```python
from build123d import *

# Parameters (mm, degrees)
SKETCH1_W             = 93.653112922
SKETCH1_H             = 50
BOSS_EXTRUDE1_DEPTH   = 2.8575
SKETCH3_W             = 23.386037641
SKETCH3_H             = 4.318
BOSS_EXTRUDE2_DEPTH   = 2.8575
CUT_EXTRUDE1_REACH    = 4.857
SKETCH4_W             = 4.572
SKETCH4_H             = 14.7575
SKETCH4_H_2           = 6.0325
CUT_EXTRUDE2_REACH    = 4.857
SKETCH5_W             = 20.574
SKETCH5_H             = 2.9845
SKETCH6_R             = 0.635
CUT_EXTRUDE3_DEPTH    = 0.127
CHAMFER1_SIZE         = 0.762
CHAMFER1_SIZE2        = 1.319822715
CHAMFER1_PART_2_SIZE  = 0.762
CHAMFER1_PART_2_SIZE2 = 1.319822715
CHAMFER1_PART_3_SIZE  = 0.762
CHAMFER1_PART_3_SIZE2 = 1.319822715
CHAMFER1_PART_4_SIZE  = 0.762
CHAMFER1_PART_4_SIZE2 = 1.319822715
CHAMFER2_SIZE         = 0.762
CHAMFER2_SIZE2        = 1.319822715
CHAMFER2_PART_2_SIZE  = 0.762
CHAMFER2_PART_2_SIZE2 = 1.319822715
CHAMFER2_PART_3_SIZE  = 0.762
CHAMFER2_PART_3_SIZE2 = 1.319822715
CHAMFER2_PART_4_SIZE  = 0.762
CHAMFER2_PART_4_SIZE2 = 1.319822715
FILLET1_R             = 0.762


with BuildPart() as part:
    # Sketch1 → Boss-Extrude1 (new body)
    with BuildSketch(Plane(origin=(0, 0, 0), x_dir=(1, 0, 0), z_dir=(0, 1, 0))):
        Rectangle(SKETCH1_W, SKETCH1_H)
    extrude(amount=BOSS_EXTRUDE1_DEPTH)

    # Sketch3 → Boss-Extrude2 (add)
    with BuildSketch(Plane.XZ):
        with Locations((-22.751037641, 27.159)):
            Rectangle(SKETCH3_W, SKETCH3_H)
        with Locations((22.751037641, 27.159)):
            Rectangle(SKETCH3_W, SKETCH3_H)
    extrude(amount=-BOSS_EXTRUDE2_DEPTH)

    # Sketch4 → Cut-Extrude1 (cut, up to next)
    with BuildSketch(Plane(origin=(0, 2.8575, 0), x_dir=(1, 0, 0), z_dir=(0, 1, 0)), mode=Mode.PRIVATE) as cut_extrude1_sk1:
        with Locations((44.540556461, 17.62125)):
            Rectangle(SKETCH4_W, SKETCH4_H)
    cut_extrude1_tool1 = extrude(cut_extrude1_sk1.sketch, amount=-CUT_EXTRUDE1_REACH, mode=Mode.PRIVATE) & part.part
    add(cut_extrude1_tool1.solids().sort_by_distance((44.540556, 2.8575, -17.62125))[0], mode=Mode.SUBTRACT)
    # Sketch4 → Cut-Extrude1 (cut, up to next)
    with BuildSketch(Plane(origin=(0, 2.8575, 0), x_dir=(1, 0, 0), z_dir=(0, 1, 0)), mode=Mode.PRIVATE) as cut_extrude1_sk2:
        with Locations((44.540556461, -21.98375)):
            Rectangle(SKETCH4_W, SKETCH4_H_2)
    cut_extrude1_tool2 = extrude(cut_extrude1_sk2.sketch, amount=-CUT_EXTRUDE1_REACH, mode=Mode.PRIVATE) & part.part
    add(cut_extrude1_tool2.solids().sort_by_distance((44.540556, 2.8575, 21.98375))[0], mode=Mode.SUBTRACT)
    # Sketch4 → Cut-Extrude1 (cut, up to next)
    with BuildSketch(Plane(origin=(0, 2.8575, 0), x_dir=(1, 0, 0), z_dir=(0, 1, 0)), mode=Mode.PRIVATE) as cut_extrude1_sk3:
        with Locations((-44.540556461, 17.62125)):
            Rectangle(SKETCH4_W, SKETCH4_H)
    cut_extrude1_tool3 = extrude(cut_extrude1_sk3.sketch, amount=-CUT_EXTRUDE1_REACH, mode=Mode.PRIVATE) & part.part
    add(cut_extrude1_tool3.solids().sort_by_distance((-44.540556, 2.8575, -17.62125))[0], mode=Mode.SUBTRACT)
    # Sketch4 → Cut-Extrude1 (cut, up to next)
    with BuildSketch(Plane(origin=(0, 2.8575, 0), x_dir=(1, 0, 0), z_dir=(0, 1, 0)), mode=Mode.PRIVATE) as cut_extrude1_sk4:
        with Locations((-44.540556461, -21.98375)):
            Rectangle(SKETCH4_W, SKETCH4_H_2)
    cut_extrude1_tool4 = extrude(cut_extrude1_sk4.sketch, amount=-CUT_EXTRUDE1_REACH, mode=Mode.PRIVATE) & part.part
    add(cut_extrude1_tool4.solids().sort_by_distance((-44.540556, 2.8575, 21.98375))[0], mode=Mode.SUBTRACT)

    # Sketch5 → Cut-Extrude2 (cut, up to next)
    with BuildSketch(Plane.XZ, mode=Mode.PRIVATE) as cut_extrude2_sk1:
        with Locations((22.225, -18.74525)):
            Rectangle(SKETCH5_W, SKETCH5_H)
    cut_extrude2_tool1 = extrude(cut_extrude2_sk1.sketch, amount=-CUT_EXTRUDE2_REACH, mode=Mode.PRIVATE) & part.part
    add(cut_extrude2_tool1.solids().sort_by_distance((22.225, 0, -18.74525))[0], mode=Mode.SUBTRACT)
    # Sketch5 → Cut-Extrude2 (cut, up to next)
    with BuildSketch(Plane.XZ, mode=Mode.PRIVATE) as cut_extrude2_sk2:
        with Locations((-22.225, -18.74525)):
            Rectangle(SKETCH5_W, SKETCH5_H)
    cut_extrude2_tool2 = extrude(cut_extrude2_sk2.sketch, amount=-CUT_EXTRUDE2_REACH, mode=Mode.PRIVATE) & part.part
    add(cut_extrude2_tool2.solids().sort_by_distance((-22.225, 0, -18.74525))[0], mode=Mode.SUBTRACT)

    # Sketch6 → Cut-Extrude3 (cut)
    with BuildSketch(Plane.XZ):
        with Locations((-25.799037641, 26.778)):
            Circle(SKETCH6_R)
        with Locations((-23.767037641, 26.778)):
            Circle(SKETCH6_R)
        with Locations((-21.735037641, 26.778)):
            Circle(SKETCH6_R)
        with Locations((-19.703037641, 26.778)):
            Circle(SKETCH6_R)
        with Locations((19.703037641, 26.778)):
            Circle(SKETCH6_R)
        with Locations((21.735037641, 26.778)):
            Circle(SKETCH6_R)
        with Locations((23.767037641, 26.778)):
            Circle(SKETCH6_R)
        with Locations((25.799037641, 26.778)):
            Circle(SKETCH6_R)
        with Locations((44.286556461, 4.3625)):
            Circle(SKETCH6_R)
        with Locations((-44.286556461, 7.4105)):
            Circle(SKETCH6_R)
        with Locations((-44.286556461, 5.3785)):
            Circle(SKETCH6_R)
        with Locations((-44.286556461, 3.3465)):
            Circle(SKETCH6_R)
        with Locations((-44.286556461, 1.3145)):
            Circle(SKETCH6_R)
    extrude(amount=-CUT_EXTRUDE3_DEPTH, mode=Mode.SUBTRACT)

    # Chamfer1
    chamfer1_edges = [part.edges().sort_by_distance(p)[0] for p in [
        (-34.444056461, 1.42875, 29.318),
    ]]
    chamfer1_side = [part.faces().sort_by_distance(p)[0] for p in [
        (-22.751037641, 1.42875, 29.318),
    ]]
    chamfer(chamfer1_edges, length=CHAMFER1_SIZE, length2=CHAMFER1_SIZE2, reference=chamfer1_side[0])

    # Chamfer1 part 2
    chamfer1_part_2_edges = [part.edges().sort_by_distance(p)[0] for p in [
        (11.05801882, 1.42875, 29.318),
    ]]
    chamfer1_part_2_side = [part.faces().sort_by_distance(p)[0] for p in [
        (22.751037641, 1.42875, 29.318),
    ]]
    chamfer(chamfer1_part_2_edges, length=CHAMFER1_PART_2_SIZE, length2=CHAMFER1_PART_2_SIZE2, reference=chamfer1_part_2_side[0])

    # Chamfer1 part 3
    chamfer1_part_3_edges = [part.edges().sort_by_distance(p)[0] for p in [
        (-46.826556461, 1.42875, 18.9675),
    ]]
    chamfer1_part_3_side = [part.faces().sort_by_distance(p)[0] for p in [
        (-46.826556461, 1.42875, 4.3625),
    ]]
    chamfer(chamfer1_part_3_edges, length=CHAMFER1_PART_3_SIZE, length2=CHAMFER1_PART_3_SIZE2, reference=chamfer1_part_3_side[0])

    # Chamfer1 part 4
    chamfer1_part_4_edges = [part.edges().sort_by_distance(p)[0] for p in [
        (46.826556461, 1.42875, -10.2425),
    ]]
    chamfer1_part_4_side = [part.faces().sort_by_distance(p)[0] for p in [
        (46.826556461, 1.42875, 4.3625),
    ]]
    chamfer(chamfer1_part_4_edges, length=CHAMFER1_PART_4_SIZE, length2=CHAMFER1_PART_4_SIZE2, reference=chamfer1_part_4_side[0])

    # Chamfer2
    chamfer2_edges = [part.edges().sort_by_distance(p)[0] for p in [
        (-11.05801882, 1.42875, 29.318),
    ]]
    chamfer2_side = [part.faces().sort_by_distance(p)[0] for p in [
        (-22.370037641, 1.42875, 29.318),
    ]]
    chamfer(chamfer2_edges, length=CHAMFER2_SIZE, length2=CHAMFER2_SIZE2, reference=chamfer2_side[0])

    # Chamfer2 part 2
    chamfer2_part_2_edges = [part.edges().sort_by_distance(p)[0] for p in [
        (34.444056461, 1.42875, 29.318),
    ]]
    chamfer2_part_2_side = [part.faces().sort_by_distance(p)[0] for p in [
        (23.132037641, 1.42875, 29.318),
    ]]
    chamfer(chamfer2_part_2_edges, length=CHAMFER2_PART_2_SIZE, length2=CHAMFER2_PART_2_SIZE2, reference=chamfer2_part_2_side[0])

    # Chamfer2 part 3
    chamfer2_part_3_edges = [part.edges().sort_by_distance(p)[0] for p in [
        (46.826556461, 1.42875, 18.9675),
    ]]
    chamfer2_part_3_side = [part.faces().sort_by_distance(p)[0] for p in [
        (46.826556461, 1.42875, 4.7435),
    ]]
    chamfer(chamfer2_part_3_edges, length=CHAMFER2_PART_3_SIZE, length2=CHAMFER2_PART_3_SIZE2, reference=chamfer2_part_3_side[0])

    # Chamfer2 part 4
    chamfer2_part_4_edges = [part.edges().sort_by_distance(p)[0] for p in [
        (-46.826556461, 1.42875, -10.2425),
    ]]
    chamfer2_part_4_side = [part.faces().sort_by_distance(p)[0] for p in [
        (-46.826556461, 1.42875, 3.9815),
    ]]
    chamfer(chamfer2_part_4_edges, length=CHAMFER2_PART_4_SIZE, length2=CHAMFER2_PART_4_SIZE2, reference=chamfer2_part_4_side[0])

    # Fillet1
    fillet1_edges = [part.edges().sort_by_distance(p)[0] for p in [
        (11.938, 1.42875, -20.2375),
        (11.938, 1.42875, -17.253),
        (32.512, 1.42875, -17.253),
        (32.512, 1.42875, -20.2375),
        (-32.512, 1.42875, -20.2375),
        (-32.512, 1.42875, -17.253),
        (-11.938, 1.42875, -17.253),
        (-11.938, 1.42875, -20.2375),
    ]]
    fillet(fillet1_edges, radius=FILLET1_R)


solid = part.part
```
The listing builds one solid part. Answer for the finished solid, in the listing's coordinates (mm). A direction names the side the tool comes from. Round coordinates to 2 decimals unless told otherwise and drop trailing zeros. Loops run counter-clockwise (first coordinate to the right, second up) from the corner with the lowest first, then second, coordinate; pieces in that order, holes last. Notation, with made-up numbers: (10, -34) - (31, -34) arc R7 cw to (31, -26) - close; hole circle Ø6 at (50, -38). An arc over 180 degrees is marked (long way). Use one line per item in the form item = value. Start each with the question number.
1. For a pull along Z with two mould halves and no side action, classify faces 6 (the face through (22, 1, -20.237)), 7 (the face through (-44, 1, 18.968)), 8 (the face through (-22, 1, -17.253)), 9 (the face through (-42.255, 1, -18)) as pulls with the +Z half, pulls with the -Z half, needs draft (parallel to the pull), parting line crosses it, or undercut.
2. The part is cut by section A-A on x = -10. Determine the outline of the cut face in (y, z).
3. Given pin 1 Ø0.6 at (x, z) = (20, 26.5) entering from -Y; pin 2 Ø1.4 at (y, z) = (2, 26) entering from +X; pin 3 Ø0.8 at (x, z) = (-44.29, 7.41) entering from -Y; pin 4 Ø1.4 at (y, z) = (1.5, 22.5) entering from -X, each flat-ended and moving along its own axis, determine where each tip first touches the part or whether it passes through.
4. Consider line 1 (X direction, y = 0.55, z = -18); line 2 (Z direction, x = -26.5, y = 0.3); line 3 (X direction, y = 0.35, z = -12.5). Determine where each line is inside the solid, lowest interval first. Write a range as [from, to].
5. A tool of negligible diameter and unlimited length cuts with its end or side. For faces 1 (the face through (-38, 1, 25)), 2 (the face through (-22, 1, -20.237)), 3 (the face through (-11.058, 1, 26)), 4 (the face through (42.255, 1, 22)), 5 (the face through (42.255, 1, -18)), from which of +Z, -Z, +X, -X, +Y, -Y can it reach the whole face along a straight path? Write none if from no direction.
6. The part is cut by section B-B on y = 0.8. Give the number of separate pieces and of enclosed holes in the cut face, then the cut area to 3 significant figures.
Geometry check:
q1.face_6 = undercut
q1.face_7 = pulls with the +Z half
q1.face_8 = undercut
q1.face_9 = needs draft
q2.outline = (0, -25) - (2.86, -25) - (2.86, 25) - (0, 25) - close
q3.pin_1 = 0
q3.pin_2 = 34.44
q3.pin_3 = 0.13
q3.pin_4 = -42.25
q4.line_1 = [-42.25, -32.51], [-11.94, 11.94], [32.51, 42.25]
q4.line_2 = [-25, -20.24], [-17.25, 29.32]
q4.line_3 = [-42.25, 42.25]
q5.face_1 = +Z, -X, +Y, -Y
q5.face_2 = +Y, -Y
q5.face_3 = +Z, +Y, -Y
q5.face_4 = +Z, +X, +Y, -Y
q5.face_5 = -Z, +X, +Y, -Y
q6.separate_pieces = 1
q6.enclosed_holes = 2
q6.area = 4,570 mm^2
